The model under review builds one solid part; all positions refer to its coordinate system, in mm. A direction names the side the tool comes from. Give positions to 0.01 mm unless a question says otherwise; leave off trailing zeros. Write each loop counter-clockwise with the first axis right and the second up, starting at its lowest first coordinate (ties: lowest second). Pieces come first, ordered by that corner, then holes. Notation, with made-up numbers: M 59,35 L 81,35 A21 ccw 81,72 Z; hole C 29.5,40.25 d3. An arc over 180 degrees is marked long. Write item = value, one per line. Start each with the question number.
Autodesk Inventor part; units mm, degrees
ref_plane "YZ Plane" through (0, 0, 0) normal (1, 0, 0) x (0, 1, 0)
ref_plane "XZ Plane" through (0, 0, 0) normal (0, 1, 0) x (-1, 0, 0)
ref_plane "XY Plane" through (0, 0, 0) normal (0, 0, 1) x (1, 0, 0)
sketch "Sketch1" plane through (0, 0, 0) normal (0, 1, 0) x (-1, 0, 0)
  line L0 (16, -28.5) -> (-16, -28.5)
  line L1 (-16, -28.5) -> (-16, 28.5)
  line L2 (-16, 28.5) -> (16, 28.5)
  line L3 (16, 28.5) -> (16, -28.5)
  line L4 (16, -28.5) -> (-16, 28.5) construction
  line L5 (-16, -28.5) -> (16, 28.5) construction
  point P0 (0, 0)
  dimension "d0" = 32
  dimension "d1" = 57
extrude "Extrusion1" add sketch "Sketch1" along normal blind 1
sketch "Sketch2" plane through (0, 1, 0) normal (0, 1, 0) x (1, 0, 0)
  line L0 (-9.5, -27.5) -> (9.5, -27.5)
  line L1 (15.5, -25.5) -> (15.5, 25.5)
  line L2 (9.5, 27.5) -> (-9.5, 27.5)
  line L3 (-15.5, 25.5) -> (-15.5, -25.5)
  line L4 (-15.5, -27.5) -> (15.5, 27.5) construction
  line L5 (15.5, -27.5) -> (-15.5, 27.5) construction
  line L6 (13.5, -25.5) -> (13.5, 25.5)
  line L7 (-13.5, 25.5) -> (-13.5, -25.5)
  line L8 (-16, -28.5) -> (16, -28.5)
  line L9 (-9.5, -28.4306) -> (-9.5, -25.5)
  line L10 (9.5, 25.5) -> (9.5, 27.5)
  line L11 (-9.5, -16.8548) -> (-9.5, 16.8548)
  line L12 (-9.5, 25.5) -> (-9.5, 28.5928)
  line L13 (9.5, -28.5) -> (9.5, -25.5)
  line L14 (9.5, -16.8548) -> (9.5, 16.8548)
  line L15 (13.5, -25.5) -> (15.5, -25.5)
  line L16 (15.5, 25.5) -> (13.5, 25.5)
  line L17 (9.5, 25.5) -> (-9.5, 25.5)
  line L18 (-13.5, 25.5) -> (-15.5, 25.5)
  line L19 (-15.5, -25.5) -> (-13.5, -25.5)
  line L20 (-9.5, -25.5) -> (9.5, -25.5)
  point P0 (0, 0)
  dimension "d4" = 31
  dimension "d5" = 55
  dimension "d6" = 2
extrude "Extrusion2" add sketch "Sketch2" along normal blind 4
sketch "Sketch3" plane through (15.5, 1, 25.5) normal (1, 0, 0) x (0, 0, -1)
  circle A0 centre (25.5, 6.5) radius 5
  line L0 (-3, 0) -> (54, 0)
  point P0 (25.5, -1)
  dimension "d11" = 10
  dimension "d12" = 6.5
extrude "Extrusion3" cut sketch "Sketch3" against normal through all
sketch "Sketch4" plane through (0, 0, 0) normal (0, -1, 0) x (1, 0, 0)
  line L0 (7.5, -7.5) -> (-7.5, -7.5)
  line L1 (-7.5, -7.5) -> (-7.5, 7.5)
  line L2 (-7.5, 7.5) -> (7.5, 7.5)
  line L3 (7.5, 7.5) -> (7.5, -7.5)
  line L4 (7.5, -7.5) -> (-7.5, 7.5) construction
  line L5 (-7.5, -7.5) -> (7.5, 7.5) construction
  point P0 (0, 0)
  dimension "d15" = 15
  dimension "d16" = 15
extrude "Extrusion4" [suppressed]
sketch "Sketch5" plane through (0, 1, 0) normal (0, 1, 0) x (1, 0, 0)
  line L0 (-13.5, -25.5) -> (-15.5, -25.5)
  line L1 (-15.5, -25.5) -> (-15.5, 25.5)
  line L2 (-15.5, 25.5) -> (-13.5, 25.5)
  line L3 (-13.5, 25.5) -> (-13.5, -25.5)
  line L4 (9.5, -27.5) -> (-9.5, -27.5)
  line L5 (-9.5, -27.5) -> (-9.5, -25.5)
  line L6 (-9.5, -25.5) -> (9.5, -25.5)
  line L7 (9.5, -25.5) -> (9.5, -27.5)
  line L8 (9.5, 27.5) -> (9.5, 25.5)
  line L9 (9.5, 25.5) -> (-9.5, 25.5)
  line L10 (-9.5, 25.5) -> (-9.5, 27.5)
  line L11 (-9.5, 27.5) -> (9.5, 27.5)
  line L12 (13.5, 25.5) -> (15.5, 25.5)
  line L13 (15.5, 25.5) -> (15.5, -25.5)
  line L14 (15.5, -25.5) -> (13.5, -25.5)
  line L15 (13.5, -25.5) -> (13.5, 25.5)
  line L16 (16, 28.5) -> (-16, 28.5)
  line L17 (-16, 28.5) -> (-16, -28.5)
  line L18 (-16, -28.5) -> (16, -28.5)
  line L19 (16, -28.5) -> (16, 28.5)
  line L20 (-8.5, -8.5) -> (8.5, -8.5)
  line L21 (8.5, -8.5) -> (8.5, 8.5)
  line L22 (8.5, 8.5) -> (-8.5, 8.5)
  line L23 (-8.5, 8.5) -> (-8.5, -8.5)
  point P0 (0, 0)
extrude "Extrusion5" [suppressed]
properties part number "hull_cover_closed"
Item 1: To check wall thickness, follow probe 1 along X at (y, z) = (3.35, -13.5); probe 2 along Z at (x, y) = (7, 4.7); probe 3 along Y at (x, z) = (10, 11). State the ranges of each line that lie inside material, in increasing order. Write a range as [from, to].
Item 2: We need section B-B, the plane x = 1.5. Write out the cut boundary in (y, z), and give its area (3 significant figures).
Item 3: For faces 1 (the flat face through (13.5, 2, 0)), 2 (the flat face through (9.5, 3, -26)), 3 (the flat face through (-15, 3, 25.5)), 4 (the flat face through (0, 3, 25.5)), list the 3-axis set-ups (+Z, -Z, +X, -X, +Y, -Y) from which the entire face can be reached by the end or side of a thin tool; tool diameter is ignored.
Item 4: We need section A-A, the plane y = 1.8. Write out the cut boundary in (x, z).
Item 5: We need section C-C, the plane y = 4.4. Write out the cut boundary in (x, z).
Item 6: We need section D-D, the plane z = -10. Write out the cut boundary in (x, y).
Item 7: The part is to be moulded in two halves that separate along X. For faces 5 (the flat face through (0, 3, -25.5)), 6 (the flat face through (0, 3, 27.5)), 7 (the flat face through (-16, 0.5, 0.4)), say which applies: released by +X, released by -X, zero draft, split by the parting line, or undercut.
Item 8: Clearance check with flat-ended pins moving along their axes: P1, Ø2, axis at x = -14, y = 4, coming from the +Z side; P2, Ø1.6, axis at y = 3.5, z = -26.5, coming from the -X side; P3, Ø2, axis at x = 1.5, y = 2.5, coming from the +Z side. State where each tip first meets the part, or that it passes through.
Worked out:
q1.probe_1 = [-15.5, -13.5], [13.5, 15.5]
q1.probe_2 = [-27.5, -25.5], [25.5, 27.5]
q1.probe_3 = [0, 1]
q2.outline = M 0,-28.5 L 1,-28.5 L 1,-27.5 L 5,-27.5 L 5,-25.5 L 1,-25.5 L 1,25.5 L 5,25.5 L 5,27.5 L 1,27.5 L 1,28.5 L 0,28.5 Z
q2.area = 73.0 mm²
q3.face_1 = +Z, -Z, +Y
q3.face_2 = +Z, -Z, +X, +Y
q3.face_3 = +Z, -X, +Y
q3.face_4 = +Y
q4.outline = M -15.5,-25.5 L -13.5,-25.5 L -13.5,25.5 L -15.5,25.5 Z; M -9.5,-27.5 L 9.5,-27.5 L 9.5,-25.5 L -9.5,-25.5 Z; M -9.5,25.5 L 9.5,25.5 L 9.5,27.5 L -9.5,27.5 Z; M 13.5,-25.5 L 15.5,-25.5 L 15.5,25.5 L 13.5,25.5 Z
q5.outline = M -15.5,-25.5 L -13.5,-25.5 L -13.5,-3.92 L -15.5,-3.92 Z; M -15.5,3.92 L -13.5,3.92 L -13.5,25.5 L -15.5,25.5 Z; M -9.5,-27.5 L 9.5,-27.5 L 9.5,-25.5 L -9.5,-25.5 Z; M -9.5,25.5 L 9.5,25.5 L 9.5,27.5 L -9.5,27.5 Z; M 13.5,-25.5 L 15.5,-25.5 L 15.5,-3.92 L 13.5,-3.92 Z; M 13.5,3.92 L 15.5,3.92 L 15.5,25.5 L 13.5,25.5 Z
q6.outline = M -16,0 L 16,0 L 16,1 L 15.5,1 L 15.5,5 L 13.5,5 L 13.5,1 L -13.5,1 L -13.5,5 L -15.5,5 L -15.5,1 L -16,1 Z
q7.face_5 = undercut
q7.face_6 = zero draft
q7.face_7 = released by -X
q8.P1 = 25.5
q8.P2 = -9.5
q8.P3 = 27.5
